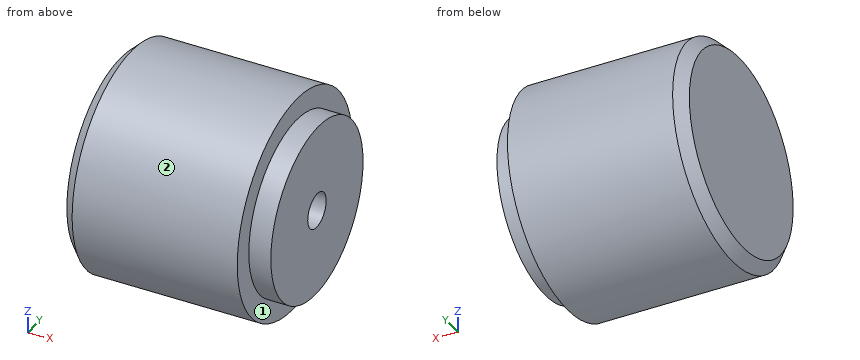
Autodesk Inventor part; units mm, degrees
ref_plane "YZ Plane" through (0, 0, 0) normal (1, 0, 0) x (0, 1, 0)
ref_plane "XZ Plane" through (0, 0, 0) normal (0, 1, 0) x (-1, 0, 0)
ref_plane "XY Plane" through (0, 0, 0) normal (0, 0, 1) x (1, 0, 0)
sketch "Sketch1" plane through (0, 0, 0) normal (0, 0, 1) x (1, 0, 0)
  line L0 (0, 0) -> (18, 0)
  line L1 (18, 0) -> (18, 10)
  line L2 (18, 10) -> (0, 10)
  line L3 (0, 10) -> (0, 0)
  line L4 (18, 0) -> (16, 0)
  line L5 (16, 0) -> (16, 8)
  line L6 (16, 8) -> (18, 8)
  line L7 (18, 8) -> (18, 0)
  line L8 (16, 8) -> (16, 10)
  dimension "d0" = 18
  dimension "d1" = 10
  dimension "d2" = 2
  dimension "d3" = 8
revolve "Revolution1" add sketch "Sketch1" angle 360 about axis through (0, 0, 0) along (1, 0, 0) contours L3 L2 L8 L5 L0 | L5 L6 L1 L0
chamfer "Chamfer1" distance 1 angle 45 1 edges at (0, -10, 0)
sketch "Sketch2" plane through (18, 0, 0) normal (1, 0, 0) x (0, 0, -1)
  point P0 (0, 0)
  point P1 (0, 0)
hole "Hole1" at (18, 0, 0) direction (-1, 0, 0) diameter 3.2 depth 14 tip angle 118
thread "Thread1"
properties part number "üllő"
CAD build for the part. Positions are in the model's coordinates, mm. Face numbers are marked on the shaded views. A direction names the side the tool comes from. Give positions to 0.01 mm unless a question says otherwise; leave off trailing zeros. Order: outer loops, then holes, each group sorted by start corner. A loop starts at its lowest first (then second) coordinate and runs counter-clockwise, first axis right, second up. Notation, with made-up numbers: (35, -15.5) -> (53, -15.5) arc R30 cw to (53, 11.5) -> close; hole circle Ø11 at (30, -27). An arc over 180 degrees is marked (long way). Return JSON: item names as keys, results as strings.
Q1. Saw through at B-B (x = 2). Write the cut outline in (y, z).
Working result:
{"outline": "circle Ø20 at (0, 0)"}
Q2. Which spindle directions (+Z, -Z, +X, -X, +Y, -Y) get a long thin tool onto all of the face, cutting with end or side? Do the marked faces 1 and 2. Say none if no direction does.
Working result:
{"face 1": "+X", "face 2": "+X, -X"}
Q3. Drill centre lines: line 1 (Z direction, x = 4, y = -6); line 2 (Z direction, x = 9, y = 7.5); line 3 (X direction, y = -4.5, z = 8). Where is each one in solid material? Low to high.
Working result:
{"line 1": "-8 to 8", "line 2": "-6.61 to 6.61", "line 3": "0.18 to 16"}
Q4. Saw through at A-A (x = 8). Write the cut outline in (y, z).
Working result:
{"outline": "circle Ø20 at (0, 0); hole circle Ø3.2 at (0, 0)"}
Q5. Flat gauge pins, fed straight in: pin 1 (5 mm diameter, centred on x = 16, y = 7.5, fed in from +Z); pin 2 (1.5 mm diameter, centred on x = 13.5, y = 7, fed in from +Z); pin 3 (1.5 mm diameter, centred on x = 7.5, y = -1.5, fed in from -Z). Where does each tip first touch, or does it go through?
Working result:
{"pin 1": "z = 8.66", "pin 2": "z = 7.81", "pin 3": "z = -9.97"}
